Check sheet for the drawn part. Datum: minimum x, y, z corner. Units: mm. Round coordinates to 2 decimals unless told otherwise and drop trailing zeros. Write each loop counter-clockwise with the first axis right and the second up, starting at its lowest first coordinate (ties: lowest second). Pieces come first, ordered by that corner, then holes. Notation, with made-up numbers: (-4.75, 38.5) - (29.25, 38.5) arc R19 cw to (29.25, 46.5) - close; hole circle Ø3 at (72, 0.5). An arc over 180 degrees is marked (long way). Return JSON: item names as keys, results as strings. Group by question number.
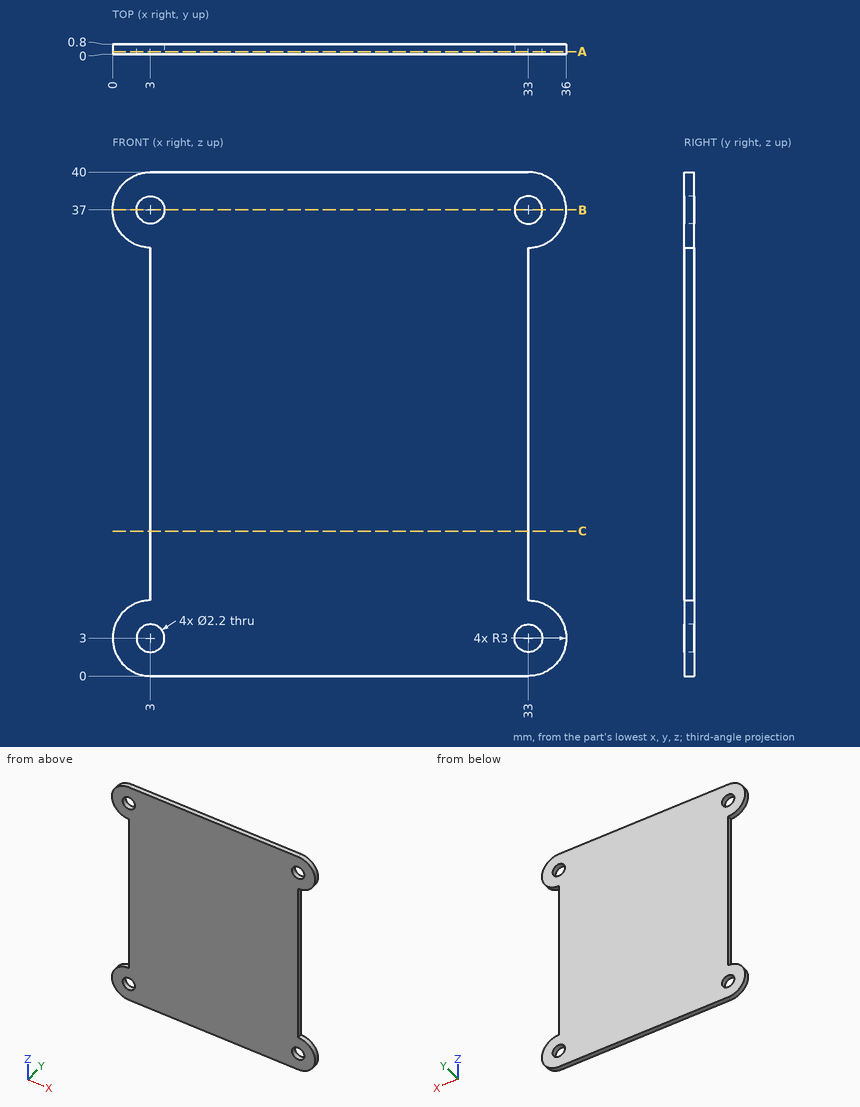
1. Section check B-B (z = 37). Enter the section's corners in (x, y).
2. Depth check by flat-ended pin: pin 1 Ø1.3 at (x, z) = (3, 37) entering from +Y. Enter the tip coordinate at first touch or a pass-through.
3. Section check A-A (y = 0.2). Enter the section's corners in (x, z).
4. Section check C-C (z = 11.5). Enter the section's corners in (x, y), and give its area (3 significant figures).
5. Material ranges on line 1 along X through (y, z) = (0.15, 37.5); line 2 along X through (y, z) = (0.5, 27), recorded low to high.
Result sheet:
{
 "1": {"outline": "(0, 0) - (1.9, 0) - (1.9, 0.8) - (0, 0.8) - close; (4.1, 0) - (31.9, 0) - (31.9, 0.8) - (4.1, 0.8) - close; (34.1, 0) - (36, 0) - (36, 0.8) - (34.1, 0.8) - close"},
 "2": {"pin 1": "passes through"},
 "3": {"outline": "(3, 0) - (33, 0) arc R3 ccw to (33, 6) - (33, 34) arc R3 ccw to (33, 40) - (3, 40) arc R3 ccw to (3, 34) - (3, 6) arc R3 ccw to start; hole circle Ø2.2 at (3, 3); hole circle Ø2.2 at (3, 37); hole circle Ø2.2 at (33, 3); hole circle Ø2.2 at (33, 37)"},
 "4": {"outline": "(3, 0) - (33, 0) - (33, 0.8) - (3, 0.8) - close", "area": "24.0 mm²"},
 "5": {"line 1": "x = 0.04 to 2.02, 3.98 to 32.02, 33.98 to 35.96", "line 2": "x = 3 to 33"}
}
